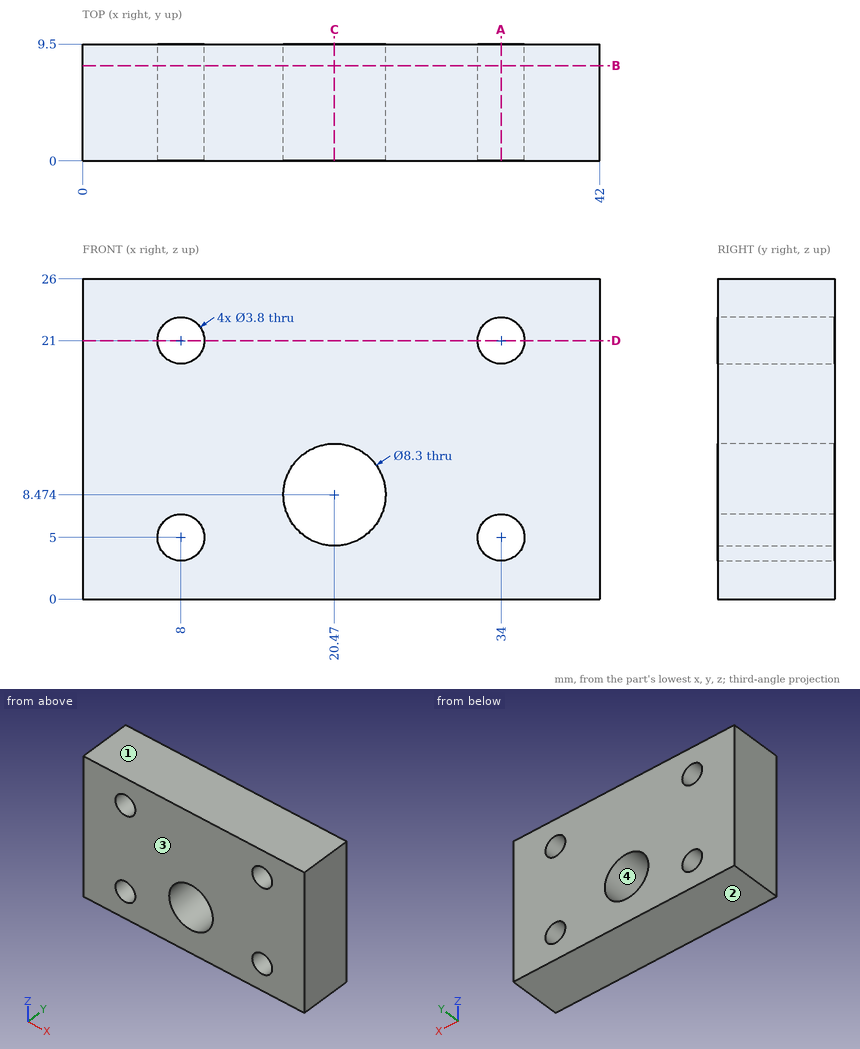
The drawing under review shows one solid part. Ordinate dimensions are in mm from its lowest x, y, z. Give positions to 0.01 mm unless a question says otherwise; leave off trailing zeros. Write each loop counter-clockwise with the first axis right and the second up, starting at its lowest first coordinate (ties: lowest second). Pieces come first, ordered by that corner, then holes.
1. Draft analysis for pull direction Z (two halves, no side actions). For the marked faces 1, 2, 3 and 4, state which applies: +Z half, -Z half, draft (parallel to the pull), parting line (faces both ways), or undercut.
2. Add section C-C, the plane x = 20.47. Write out the cut boundary in (y, z), plus the area to 3 significant figures.
3. Add section A-A, the plane x = 34. Write out the cut boundary in (y, z).
4. Wall thickness on L1, parallel to X at y = 6.75, z = 21; L2, parallel to X at y = 2.25, z = 5; L3, parallel to X at y = 3.5, z = 21.75 (1 decimal): over which ranges is each line inside the solid? List them lowest first.
5. Add section D-D, the plane z = 21. Write out the cut boundary in (x, y), plus the area to 3 significant figures.
6. Add section B-B, the plane y = 7.75. Write out the cut boundary in (x, z).
Worked answers:
1. face 1: +Z half
1. face 2: -Z half
1. face 3: draft
1. face 4: undercut
2. outline: (0, 0) - (9.5, 0) - (9.5, 4.32) - (0, 4.32) - close; (0, 12.62) - (9.5, 12.62) - (9.5, 26) - (0, 26) - close
2. area: 168 mm2
3. outline: (0, 0) - (9.5, 0) - (9.5, 3.1) - (0, 3.1) - close; (0, 6.9) - (9.5, 6.9) - (9.5, 19.1) - (0, 19.1) - close; (0, 22.9) - (9.5, 22.9) - (9.5, 26) - (0, 26) - close
4. L1: x = 0 to 6.1, 9.9 to 32.1, 35.9 to 42
4. L2: x = 0 to 6.1, 9.9 to 18.2, 22.74 to 32.1, 35.9 to 42
4. L3: x = 0 to 6.3, 9.7 to 32.3, 35.7 to 42
5. outline: (0, 0) - (6.1, 0) - (6.1, 9.5) - (0, 9.5) - close; (9.9, 0) - (32.1, 0) - (32.1, 9.5) - (9.9, 9.5) - close; (35.9, 0) - (42, 0) - (42, 9.5) - (35.9, 9.5) - close
5. area: 327 mm2
6. outline: (0, 0) - (42, 0) - (42, 26) - (0, 26) - close; hole circle Ø3.8 at (8, 5); hole circle Ø3.8 at (8, 21); hole circle Ø8.3 at (20.47, 8.47); hole circle Ø3.8 at (34, 5); hole circle Ø3.8 at (34, 21)
